Part print with two shaded views. Sizes in mm from the minimum x, y, z corner. A direction names the side the tool comes from. Round coordinates to 2 decimals unless told otherwise and drop trailing zeros. Write each loop counter-clockwise with the first axis right and the second up, starting at its lowest first coordinate (ties: lowest second). Pieces come first, ordered by that corner, then holes. Notation, with made-up numbers: (46, -11.5) - (73, -11.5) arc R18 ccw to (73, 10.5) - close; hole circle Ø7 at (69, 88). An arc over 180 degrees is marked (long way). Use one line per item in the form item = value. Start each with the question number.
Item 1: Pull direction Z, two halves, no side cores. Call the marked faces 4, 5 and 6: +Z half, -Z half, draft (parallel to the pull), parting line (faces both ways), or undercut.
Item 2: Band-saw the part on B-B, the plane y = 6.35. List the corners of the cut face in (x, z), and give its area (3 significant figures).
Item 3: Tool access for the marked faces 1, 2 and 3: list every direction of +Z, -Z, +X, -X, +Y, -Y with a clear straight run to the whole face (end or side of a thin tool).
Item 4: Band-saw the part on C-C, the plane x = 8.75. List the corners of the cut face in (y, z), and give its area (3 significant figures).
Item 5: Pin check, flat tips, straight feed: pin 1 (3 mm diameter, centred on x = 8, y = 24, fed in from -Z); pin 2 (4 mm diameter, centred on y = 15, z = 9, fed in from -X); pin 3 (4 mm diameter, centred on y = 25.5, z = 5, fed in from +X) (3 decimals). Stop position of each tip, or through.
Item 6: Drill centre lines: L1, parallel to Z at x = 13, y = 44.45; L2, parallel to Y at x = 11.5, z = 9.5; L3, parallel to Y at x = 8.75, z = 9.5. Where is each one in solid material? Low to high.
Item 7: Band-saw the part on A-A, the plane z = 9.5. List the corners of the cut face in (x, y).
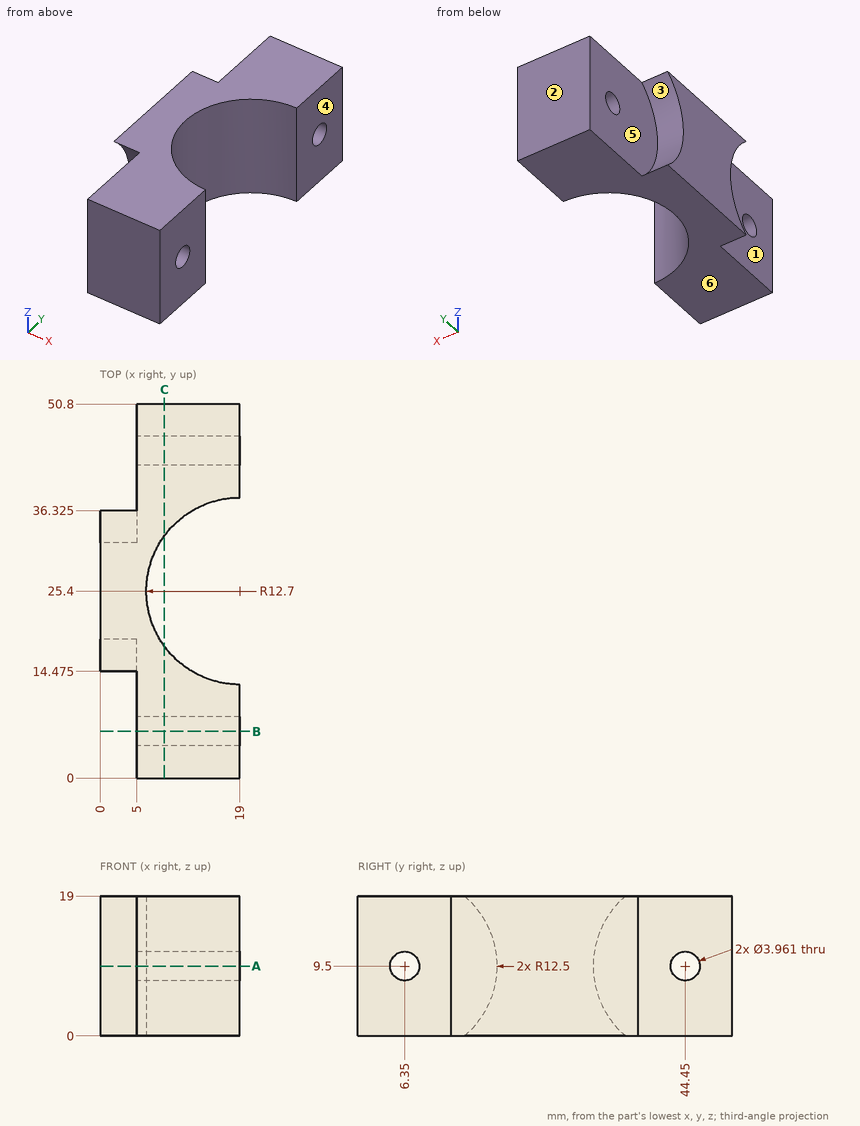
Determined:
q1.face_4 = draft
q1.face_5 = undercut
q1.face_6 = -Z half
q2.outline = (5, 0) - (19, 0) - (19, 7.52) - (5, 7.52) - close; (5, 11.48) - (19, 11.48) - (19, 19) - (5, 19) - close
q2.area = 211 mm²
q3.face_1 = -X, -Y
q3.face_2 = +Z, -Z, +X, -X, +Y
q3.face_3 = -X, +Y
q4.outline = (0, 0) - (17.9, 0) - (17.9, 19) - (0, 19) - close; (32.9, 0) - (50.8, 0) - (50.8, 19) - (32.9, 19) - close; hole circle Ø3.96 at (6.35, 9.5); hole circle Ø3.96 at (44.45, 9.5)
q4.area = 656 mm²
q5.pin_1 = through
q5.pin_2 = 5
q5.pin_3 = 6.475
q6.L1 = 0 to 7.52, 11.48 to 19
q6.L2 = 0 to 4.37, 8.33 to 15.15, 35.65 to 42.47, 46.43 to 50.8
q6.L3 = 0 to 4.37, 8.33 to 17.9, 32.9 to 42.47, 46.43 to 50.8
q7.outline = (0, 18.85) - (5, 18.85) - (5, 8.33) - (19, 8.33) - (19, 12.7) arc R12.7 cw to (19, 38.1) - (19, 42.47) - (5, 42.47) - (5, 31.95) - (0, 31.95) - close; (5, 0) - (19, 0) - (19, 4.37) - (5, 4.37) - close; (5, 46.43) - (19, 46.43) - (19, 50.8) - (5, 50.8) - close
